Source: CAD feature listing. Evaluate the final solid. Frame: model axes, mm. Face numbers are marked on the shaded views. A direction names the side the tool comes from. Round coordinates to 2 decimals unless told otherwise and drop trailing zeros. Write each loop counter-clockwise with the first axis right and the second up, starting at its lowest first coordinate (ties: lowest second). Pieces come first, ordered by that corner, then holes. Notation, with made-up numbers: (37, -28.5) -> (83, -28.5) arc R30 cw to (83, 6.5) -> close; hole circle Ø6 at (76, 71). An arc over 180 degrees is marked (long way). Put each result on its own line as item: value.
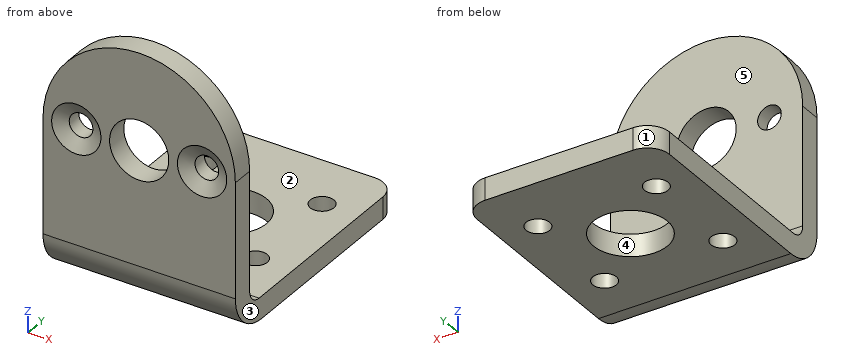
```python
from build123d import *
from OCP.BRepFilletAPI import BRepFilletAPI_MakeChamfer

# Parameters (mm, degrees)
EXTRUDE_1_DEPTH     = 3
SKETCH_2_R          = 4
SKETCH_2_R_2        = 1.6
CUT_EXTRUDE_1_DEPTH = 5
SKETCH_3_W          = 26
SKETCH_3_H          = 3
EXTRUDE_2_DEPTH     = 31
FILLET_1_R          = 2
FILLET_2_R          = 5.5
SKETCH_4_R          = 5
SKETCH_4_R_2        = 1.6
CUT_EXTRUDE_2_DEPTH = 31
FILLET_3_R          = 3
CHAMFER_1_SIZE      = 1
CHAMFER_1_SIZE2     = 1.732050808


with BuildPart() as part:
    # Sketch 1 → Extrude 1 (new body)
    with BuildSketch(Plane(origin=(0, 0, 0), x_dir=(1, 0, 0), z_dir=(0, 1, 0))):
        with BuildLine():
            Line((13, 0), (-13, 0))
            ThreePointArc((-13, 0), (0, -13), (13, 0))
        make_face()
        with BuildLine():
            ThreePointArc((13, 0), (0, 13), (-13, 0))
            Line((-13, 0), (13, 0))
        make_face()
        with BuildLine():
            Line((-13, 21), (-13, 0))
            ThreePointArc((-13, 0), (0, 13), (13, 0))
            Line((13, 0), (13, 21))
            Line((13, 21), (-13, 21))
        make_face()
    extrude(amount=EXTRUDE_1_DEPTH)

    # Sketch 2 → Cut-Extrude 1 (cut)
    with BuildSketch(Plane(origin=(0, 3, 0), x_dir=(1, 0, 0), z_dir=(0, 1, 0))):
        with Locations(Location((0, 0, 0), (0, 0, 270))):
            Circle(SKETCH_2_R)
        with Locations(Location((-8.5, 0, 0), (0, 0, 270))):
            Circle(SKETCH_2_R_2)
        with Locations(Location((8.5, 0, 0), (0, 0, 270))):
            Circle(SKETCH_2_R_2)
    extrude(amount=-CUT_EXTRUDE_1_DEPTH, mode=Mode.SUBTRACT)

    # Sketch 3 → Extrude 2 (add)
    with BuildSketch(Plane(origin=(0, 3, 0), x_dir=(1, 0, 0), z_dir=(0, 1, 0))):
        with Locations((0, 19.5)):
            Rectangle(SKETCH_3_W, SKETCH_3_H)
    extrude(amount=EXTRUDE_2_DEPTH)

    # Fillet 1
    fillet_1_edges = [part.edges().sort_by_distance(p)[0] for p in [
        (0, 3, -18),
    ]]
    fillet(fillet_1_edges, radius=FILLET_1_R)

    # Fillet 2
    fillet_2_edges = [part.edges().sort_by_distance(p)[0] for p in [
        (0, 0, -21),
    ]]
    fillet(fillet_2_edges, radius=FILLET_2_R)

    # Sketch 4 → Cut-Extrude 2 (cut)
    with BuildSketch(Plane(origin=(0, 0, -21), x_dir=(-1, 0, 0), z_dir=(0, 0, -1))):
        with Locations((0, 19)):
            Circle(SKETCH_4_R)
        with Locations((-8, 26)):
            Circle(SKETCH_4_R_2)
        with Locations((8, 26)):
            Circle(SKETCH_4_R_2)
        with Locations((-8, 12)):
            Circle(SKETCH_4_R_2)
        with Locations((8, 12)):
            Circle(SKETCH_4_R_2)
    extrude(amount=-CUT_EXTRUDE_2_DEPTH, mode=Mode.SUBTRACT)

    # Fillet 3
    fillet_3_edges = [part.edges().sort_by_distance(p)[0] for p in [
        (-13, 34, -19.5),
        (13, 34, -19.5),
    ]]
    fillet(fillet_3_edges, radius=FILLET_3_R)

    # Chamfer 1: one chamfer whose edges measure the first distance from different faces: ONE call of the kernel's chamfer builder (chamfer() names one face for all edges)
    chamfer_1_edges_1 = [part.edges().sort_by_distance(p)[0] for p in [
        (8.5, 0, -1.6),
    ]]
    chamfer_1_side_1 = [part.faces().sort_by_distance(p)[0] for p in [
        (8.5, 1.5, -1.6),
    ]]
    chamfer_1_edges_2 = [part.edges().sort_by_distance(p)[0] for p in [
        (-8.5, 0, -1.6),
    ]]
    chamfer_1_side_2 = [part.faces().sort_by_distance(p)[0] for p in [
        (-8.5, 1.5, -1.6),
    ]]
    chamfer_1 = BRepFilletAPI_MakeChamfer(part.part.solid().wrapped)
    for e in chamfer_1_edges_1:
        chamfer_1.Add(CHAMFER_1_SIZE, CHAMFER_1_SIZE2, e.wrapped, chamfer_1_side_1[0].wrapped)  # the first distance lies on this face
    for e in chamfer_1_edges_2:
        chamfer_1.Add(CHAMFER_1_SIZE, CHAMFER_1_SIZE2, e.wrapped, chamfer_1_side_2[0].wrapped)  # the first distance lies on this face
    add(Compound.cast(chamfer_1.Shape()), mode=Mode.REPLACE)


solid = part.part
```
Q1. Draft query along Y for the marked faces 3, 4 and 5. Return one class per face: +Y half, -Y half, draft (parallel to the pull), parting line (faces both ways), or undercut.
Ans:
face 3: draft
face 4: undercut
face 5: +Y half
Q2. Cut plane C-C on y = 26. Output: boundary loops of the cut face in (x, z), and give its area (3 significant figures).
Ans:
outline: (-13, -21) -> (-9.6, -21) -> (-9.6, -18) -> (-13, -18) -> close; (-6.4, -21) -> (6.4, -21) -> (6.4, -18) -> (-6.4, -18) -> close; (9.6, -21) -> (13, -21) -> (13, -18) -> (9.6, -18) -> close
area: 58.8 mm^2
Q3. Pin query (flat end, axial travel): pin 1 (3 mm diameter, centred on x = -8.5, z = 0, fed in from -Y); pin 2 (1.5 mm diameter, centred on x = 8.5, y = 17.5, fed in from +Z); pin 3 (3.5 mm diameter, centred on x = 8.5, z = 0, fed in from +Y). Return the tip coordinate at first contact, or that it passes through.
Ans:
pin 1: passes through
pin 2: stops at z = -18
pin 3: stops at y = 3
Q4. Reachability of the marked faces 1 and 2 from +Z, -Z, +X, -X, +Y, -Y: full face, straight path, thin tool, end or side. Return the list, or none.
Ans:
face 1: +Z, -Z, -X, +Y
face 2: +Z, +X, -X, +Y
Q5. Material intervals for line 1 (Y direction, x = 8, z = -18.8); line 2 (Y direction, x = 8, z = -18.9); line 3 (Y direction, x = 2, z = 4.5), sorted ascending. Write a range as [from, to].
Ans:
line 1: y = [1.1, 10.4], [13.6, 24.4], [27.6, 34]
line 2: y = [1.18, 10.4], [13.6, 24.4], [27.6, 34]
line 3: y = [0, 3]
Q6. Cut plane D-D on x = 8.5. Output: boundary loops of the cut face in (y, z), and give its area (3 significant figures).
Ans:
outline: (0, -15.5) arc R5.5 ccw to (5.5, -21) -> (10.48, -21) -> (10.48, -18) -> (5, -18) arc R2 cw to (3, -16) -> (3, -1.6) -> (1, -1.6) -> (0, -3.33) -> close; (0, 3.33) -> (1, 1.6) -> (3, 1.6) -> (3, 9.84) -> (0, 9.84) -> close; (13.52, -21) -> (24.48, -21) -> (24.48, -18) -> (13.52, -18) -> close; (27.52, -21) -> (34, -21) -> (34, -18) -> (27.52, -18) -> close
area: 150 mm^2
Q7. Cut plane A-A on y = 19. Output: boundary loops of the cut face in (x, z), and give its area (3 significant figures).
Ans:
outline: (-13, -21) -> (-5, -21) -> (-5, -18) -> (-13, -18) -> close; (5, -21) -> (13, -21) -> (13, -18) -> (5, -18) -> close
area: 48.0 mm^2
Q8. Cut plane B-B on x = 0. Output: boundary loops of the cut face in (y, z).
Ans:
outline: (0, -15.5) arc R5.5 ccw to (5.5, -21) -> (14, -21) -> (14, -18) -> (5, -18) arc R2 cw to (3, -16) -> (3, -4) -> (0, -4) -> close; (0, 4) -> (3, 4) -> (3, 13) -> (0, 13) -> close; (24, -21) -> (34, -21) -> (34, -18) -> (24, -18) -> close
